Autodesk Inventor part; units mm, degrees
ref_plane "YZ Plane" through (0, 0, 0) normal (1, 0, 0) x (0, 1, 0)
ref_plane "XZ Plane" through (0, 0, 0) normal (0, 1, 0) x (-1, 0, 0)
ref_plane "XY Plane" through (0, 0, 0) normal (0, 0, 1) x (1, 0, 0)
sketch "Boceto2" plane through (0, 0, 0) normal (0, 0, 1) x (1, 0, 0)
  line L0 (-6, 9) -> (-6.5, 10)
  line L1 (-6.5, 10) -> (-6.5, 16)
  line L2 (-6.5, 16) -> (-7, 16)
  line L3 (-7, 16) -> (-7, 20)
  line L4 (-7, 20) -> (-11, 20)
  line L5 (-11, 20) -> (-11, 7)
  line L6 (-11, 7) -> (-32, 7)
  line L7 (-32, 7) -> (-32, 20)
  line L8 (-32, 20) -> (-35, 24)
  line L9 (-35, 34) -> (-38, 34)
  line L10 (-38, 34) -> (-38, 15)
  line L11 (-38, 15) -> (-35.5, 15)
  line L12 (-35.5, 12) -> (-38, 12)
  line L13 (-38, 10) -> (-35.5, 10)
  line L14 (-35.5, 7) -> (-38, 7)
  line L15 (-38, 5) -> (-36, 5)
  line L16 (-36, 5) -> (-36, 3.5)
  line L17 (-36, 3.5) -> (-34.2, 3.5)
  line L18 (-34.2, 3.5) -> (-34.2, 1.5)
  line L19 (-34.2, 1.5) -> (-36, 1.5)
  line L20 (-36, 1.5) -> (-36, 0)
  line L21 (-6, 9) -> (-6, 0)
  line L22 (-36, 0) -> (-6, 0)
  line L23 (-35.5, 10) -> (-35.5, 7)
  line L24 (-38, 12) -> (-38, 10)
  line L25 (-35, 34) -> (-35, 24)
  line L26 (-35.5, 15) -> (-35.5, 12)
  line L27 (0, -6.8) -> (0, 40.8)
  line L28 (-38, 7) -> (-38, 5)
  point P0 (0, 0)
  dimension "d2" = 9
  dimension "d3" = 1
  dimension "d4" = 0.5
  dimension "d5" = 0.5
  dimension "d6" = 6
  dimension "d7" = 4
  dimension "d8" = 4
  dimension "d9" = 7
  dimension "d16" = 1.5
  dimension "d17" = 1.8
  dimension "d19" = 2
  dimension "d20" = 1.5
  dimension "d21" = 2
  dimension "d23" = 3
  dimension "d24" = 2
  dimension "d25" = 3
  dimension "d33" = 38
  dimension "d35" = 6
  dimension "d38" = 4
  dimension "d39" = 21
  dimension "d40" = 13
  dimension "d42" = 2.5
  dimension "d43" = 3
  dimension "d44" = 2.5
  dimension "d49" = 2
  dimension "d51" = 10
revolve "Revolución1" add sketch "Boceto2" angle 360 about axis through (0, -10, 0) along (0, 1, 0)
sketch "Boceto3" plane through (0, 7, 0) normal (0, 1, 0) x (1, 0, 0)
  line L0 (-0.0776, -21.9999) -> (-19.0136, 11.0671) construction
  line L1 (-19.0136, 11.0671) -> (19.0912, 10.9327) construction
  line L2 (19.0912, 10.9327) -> (-0.0776, -21.9999) construction
  circle A0 centre (0, 0) radius 11 construction
  circle A1 centre (0, 0) radius 11
  circle A2 centre (-0.0776, -21.9999) radius 2.5
  circle A3 centre (19.0912, 10.9327) radius 2.5
  circle A4 centre (-19.0136, 11.0671) radius 2.5
  dimension "d56" = 5
extrude "Extrusión1" cut sketch "Boceto3" against normal up to surface (7 mm away) contours A2 | A3 | A4
properties part number "PARTE_SUPERIOR_IGNICION"
Here's how the part is built. I have some questions about the finished solid (model axes, mm). A direction names the side the tool comes from. Coordinates: 2 decimals unless noted, no trailing zeros. Loops run counter-clockwise (first coordinate to the right, second up) from the corner with the lowest first, then second, coordinate; pieces in that order, holes last. Notation, with made-up numbers: M 80.25,24 L 104.25,24 A28 cw 104.25,54 Z; hole C 27.5,-4 d3. An arc over 180 degrees is marked long. One line per item, written item: value.
1. Imagine slicing it at A-A (y = 14). List the corners of the cut face in (x, z) for me.
Geometry says:
outline: C 0,0 d71; C 0,0 d22; hole C 0,0 d64; hole C 0,0 d13
2. Thinking about a two-plate mould opening in Z: for faces 1 (the flat face through (-32, 3.5, -13)), 2 (the cylindrical face through (-17.535, 10.986, 33.713)), 3 (the cylindrical face through (6.94, 13.59, -31.24)), which applies, +Z half, -Z half, draft (parallel to the pull), parting line (faces both ways), or undercut?
Geometry says:
face 1: draft
face 2: parting line
face 3: undercut
3. On a 3-axis mill with a long thin cutter (end or side, diameter ignored), from which of +Z, -Z, +X, -X, +Y, -Y can I reach the whole of each face in a straight line? I mean faces 4 (the cylindrical face through (5.158, 13.042, -3.955)), 5 (the cylindrical face through (4.686, 0.74, -35.694)), 6 (the cylindrical face through (7.696, 8.479, 34.656)), 7 (the cylindrical face through (-17.535, 24.367, 33.713)). Say none if no direction works.
Geometry says:
face 4: +Y
face 5: -Y
face 6: none
face 7: +Y, -Y
4. Imagine slicing it at B-B (x = 0). State how many separate pieces and enclosed holes the cut face has, and give its area (3 significant figures).
Geometry says:
separate pieces: 3
enclosed holes: 0
area: 723 mm2
5. Will these pins go through, and if not, where does the flat tip stop? pin 1 Ø6 at (x, z) = (-19.01, -11.07) entering from +Y; pin 2 Ø8 at (x, y) = (20, 19) entering from +Z; pin 3 Ø6 at (y, z) = (14, 12) entering from +X.
Geometry says:
pin 1: stops at y = 7
pin 2: stops at z = 34.47
pin 3: stops at x = 36.88
6. Imagine slicing it at D-D (y = 26). List the corners of the cut face in (x, z) for me.
Geometry says:
outline: C 0,0 d76; hole C 0,0 d70
7. Please list where these lines run through material, in increasing order: probe 1 along Z at (x, y) = (0, 10.5); probe 2 along Z at (x, y) = (0, 5.75); probe 3 along Z at (x, y) = (0, 18.2).
Geometry says:
probe 1: z = -38 to -32, -11 to -6.5, 6.5 to 11, 32 to 38
probe 2: z = -38 to -6, 6 to 19.5, 24.5 to 38
probe 3: z = -38 to -32, -11 to -7, 7 to 11, 32 to 38
